```python
from build123d import *

# Parameters (mm, degrees)
SKETCH1_W           = 45
SKETCH1_H           = 20
BOSS_EXTRUDE1_DEPTH = 1
SKETCH2_R           = 8
BOSS_EXTRUDE2_DEPTH = 12
BOSS_EXTRUDE4_DEPTH = 3.5
SKETCH4_R           = 7
CUT_EXTRUDE1_DEPTH  = 8
SKETCH8_W           = 6
SKETCH8_H           = 3
SKETCH8_W_2         = 3
SKETCH8_H_2         = 6.5
BOSS_EXTRUDE5_DEPTH = 1
SKETCH9_W           = 12.7
SKETCH9_H           = 5
BOSS_EXTRUDE6_DEPTH = 4
SKETCH10_R          = 0.5
BOSS_EXTRUDE7_DEPTH = 8


with BuildPart() as part:
    # Sketch1 → Boss-Extrude1 (new body)
    with BuildSketch(Plane.XY):
        Rectangle(SKETCH1_W, SKETCH1_H)
    extrude(amount=BOSS_EXTRUDE1_DEPTH)

    # Sketch2 → Boss-Extrude2 (add)
    with BuildSketch(Plane.XY.offset(1)):
        with Locations((13, 0)):
            Circle(SKETCH2_R)
        with Locations((-13, 0)):
            Circle(SKETCH2_R)
    extrude(amount=BOSS_EXTRUDE2_DEPTH)

    # Sketch3 → Boss-Extrude4 (add)
    with BuildSketch(Plane.XY.offset(1)):
        with BuildLine():
            Line((-3.5, 6.5), (3.5, 6.5))
            ThreePointArc((3.5, 6.5), (5, 8), (3.5, 9.5))
            Line((3.5, 9.5), (-3.5, 9.5))
            ThreePointArc((-3.5, 9.5), (-5, 8), (-3.5, 6.5))
        make_face()
    extrude(amount=BOSS_EXTRUDE4_DEPTH)

    # Sketch4 → Cut-Extrude1 (cut)
    with BuildSketch(Plane.XY.offset(13)):
        with Locations((-13, 0)):
            Circle(SKETCH4_R)
        with Locations((13, 0)):
            Circle(SKETCH4_R)
    extrude(amount=-CUT_EXTRUDE1_DEPTH, mode=Mode.SUBTRACT)

    # Sketch8 → Boss-Extrude5 (add)
    with BuildSketch(Plane(origin=(0, 0, 0), x_dir=(-1, 0, 0), z_dir=(0, 0, -1))):
        Rectangle(SKETCH8_W, SKETCH8_H)
        with Locations((-19.5, 0)):
            Rectangle(SKETCH8_W, SKETCH8_H)
        with Locations((18.449397774, 0)):
            Rectangle(SKETCH8_W_2, SKETCH8_H_2)
    extrude(amount=BOSS_EXTRUDE5_DEPTH)

    # Sketch9 → Boss-Extrude6 (add)
    with BuildSketch(Plane(origin=(0, 0, 0), x_dir=(-1, 0, 0), z_dir=(0, 0, -1))):
        with Locations((0, -7.5)):
            Rectangle(SKETCH9_W, SKETCH9_H)
    extrude(amount=BOSS_EXTRUDE6_DEPTH)

    # Sketch10 → Boss-Extrude7 (add)
    with BuildSketch(Plane.XZ.offset(10)):
        with Locations((-3.85, -2.098004041)):
            Circle(SKETCH10_R)
        with Locations((-1.31, -2.098004041)):
            Circle(SKETCH10_R)
        with Locations((1.23, -2.098004041)):
            Circle(SKETCH10_R)
        with Locations((3.77, -2.098004041)):
            Circle(SKETCH10_R)
    extrude(amount=BOSS_EXTRUDE7_DEPTH)


solid = part.part
```
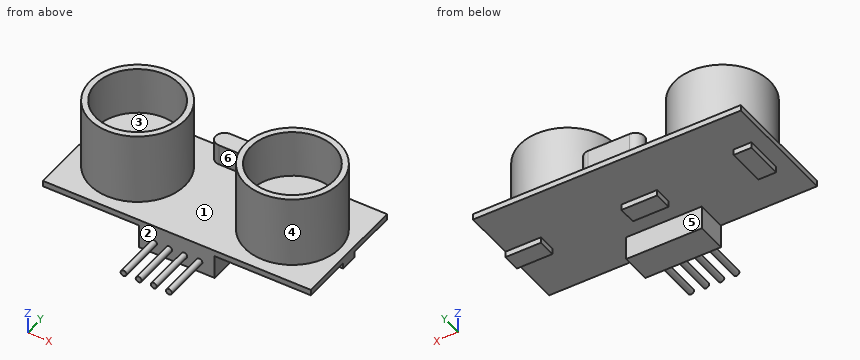
Here's how the part is built. I have some questions about the finished solid (model axes, mm). Face numbers are marked on the shaded views. A direction names the side the tool comes from. Round coordinates to 2 decimals unless told otherwise and drop trailing zeros. Order: outer loops, then holes, each group sorted by start corner. A loop starts at its lowest first (then second) coordinate and runs counter-clockwise, first axis right, second up. Notation, with made-up numbers: M 53,63.25 L 59,63.25 A10 cw 59,74.25 Z; hole C 65.5,-38.75 d3. An arc over 180 degrees is marked long. Use CSV: the item, a comma, the result in double quotes.
1) I want a section at B-B (x = 2.5). List the corners of the cut face in (y, z) for me, then the cut area to 3 significant figures.
Taken from the geometry:
outline,"M -10,-4 L -5,-4 L -5,0 L -1.5,0 L -1.5,-1 L 1.5,-1 L 1.5,0 L 10,0 L 10,1 L 9.5,1 L 9.5,4.5 L 6.5,4.5 L 6.5,1 L -10,1 Z"
area,"53.5 mm^2"
2) If we mould it in two halves opening along Y, with no side actions, what happens to the marked faces 1, 2 and 3? For each: pulls with the +Y half, pulls with the -Y half, needs draft (parallel to the pull), parting line crosses it, or undercut.
Taken from the geometry:
face 1,"needs draft"
face 2,"pulls with the -Y half"
face 3,"undercut"
3) I want a section at C-C (z = 2.5). List the corners of the cut face in (x, y) for me.
Taken from the geometry:
outline,"C -13,0 d16; M -3.5,6.5 L 3.5,6.5 A1.5 ccw 3.5,9.5 L -3.5,9.5 A1.5 ccw Z; C 13,0 d16"
4) I'm going to push flat-ended pins straight in: P1, Ø4.5, axis at x = -3, z = -1.5, coming from the +Y side; P2, Ø2, axis at x = 2.5, y = 3.5, coming from the -Z side; P3, Ø0.5, axis at x = -18, z = -0.5, coming from the +Y side; P4, Ø8, axis at x = -15.5, z = 4, coming from the -Y side. Where does each tip first touch, or does it pass through?
Taken from the geometry:
P1,"y = 10"
P2,"z = 0"
P3,"y = 3.25"
P4,"y = -10"
5) I need wall thicknesses on line 1 along Y through (x, z) = (-13, 7); line 2 along X through (y, z) = (2, 7.5); line 3 along X through (y, z) = (-4, 8). Which ranges of each line are inside material? Lowest first, please. Write a range as [from, to].
Taken from the geometry:
line 1,"[-8, -7], [7, 8]"
line 2,"[-20.75, -19.71], [-6.29, -5.25], [5.25, 6.29], [19.71, 20.75]"
line 3,"[-19.93, -18.74], [-7.26, -6.07], [6.07, 7.26], [18.74, 19.93]"
6) On a 3-axis mill with a long thin cutter (end or side, diameter ignored), from which of +Z, -Z, +X, -X, +Y, -Y can I reach the whole of each face in a straight line? I mean the marked faces 4, 5 and 6. Say none if no direction works.
Taken from the geometry:
face 4,"+Z"
face 5,"-Z, +X, -X"
face 6,"+Z, -Y"
7) I want a section at A-A (z = 8.5). List the corners of the cut face in (x, y) for me, then the cut area to 3 significant figures.
Taken from the geometry:
outline,"C -13,0 d16; C 13,0 d16; hole C -13,0 d14; hole C 13,0 d14"
area,"94.2 mm^2"
